Design review of the part built by this model. Coordinates are the model's own, in mm. A direction names the side the tool comes from. Coordinates: 2 decimals unless noted, no trailing zeros. Write item = value, one per line. Start each with the question number.
from build123d import *

# Parameters (mm, degrees)
F1_DEPTH     = 6
F3_DEPTH     = 5
F4_R         = 2.5
F5_DEPTH     = 28.0010001
F4_R_2       = 5
F6_DEPTH     = 6
F7_R         = 5
F8_DEPTH     = 7.7510001
F9_R         = 4.5
F10_DEPTH    = 1
F11_DEPTH    = 28.0010001
F12_T1_DEPTH = 5
F12_T3_DEPTH = 5.25
F13_R        = 0.5
F14_R        = 6
F14_R_2      = 4.5
F15_DEPTH    = 1.5


# Not quite as in the source:
# - a fillet or chamfer that OpenCascade refuses, or shapes differently, is made with other operations: its cross-section is extruded or revolved along the edge and cut away or added
# - a feature names something its author has since deleted; it is built from what else it names


with BuildPart() as f1:
    # F0 (on Top) → F1 (new body, symmetric)
    with BuildSketch(Plane.XY):
        with BuildLine():
            ThreePointArc((-3.75, -10.34105894), (1.2840732714, 10.9247954596), (1.25, -10.9287464972))
            Line((1.25, -10.9287464972), (1.25, -23.9287464972))
            Line((1.25, -23.9287464972), (6.25, -23.9287464972))
            Line((6.25, -23.9287464972), (6.25, -16.9424782941))
            add(Edge.make_bspline(
                [(13.9325423216, -1.3726851266), (12.6381972805, -10.4814385995), (6.7273111737, -10.6028057635), (6.25, -16.9424782941)],
                knots=[0, 0, 0, 0, 17.3620251065, 17.3620251065, 17.3620251065, 17.3620251065], degree=3))
            ThreePointArc((13.9325423216, -1.3726851266), (0.6871708294, 13.9831254107), (-14, 0))
            Line((-14, 0), (-14, -23.9287464972))
            Line((-14, -23.9287464972), (-3.75, -23.9287464972))
            Line((-3.75, -23.9287464972), (-3.75, -10.34105894))
        make_face()
    extrude(amount=F1_DEPTH, both=True)

    # F2 (on face) → F3 (join)
    with BuildSketch(Plane(origin=(-14, 0, 0), x_dir=(0, -1, 0), z_dir=(-1, 0, 0))):
        with BuildLine():
            ThreePointArc((35.9287464972, -6), (43.7069210902, -2.7781745931), (46.9287464972, 5))
            ThreePointArc((46.9287464972, 5), (38.4000033429, 15.7188100833), (26.0391302058, 9.8161695992))
            add(Edge.make_bspline(
                [(25.4869740085, 8.4596802299), (25.6594735822, 8.8218641875), (25.8423553432, 9.2659041852), (26.0391302058, 9.8161695992)],
                knots=[0.8880126886, 0.8880126886, 0.8880126886, 0.8880126886, 1, 1, 1, 1], degree=3))
            ThreePointArc((25.4869740085, 8.4596802299), (27.0108856963, -1.4398570431), (35.9287464972, -6))
        make_face()
        with BuildLine():
            add(Edge.make_bspline(
                [(25.4869740085, 8.4596802299), (25.6594735822, 8.8218641875), (25.8423553432, 9.2659041852), (26.0391302058, 9.8161695992)],
                knots=[0.8880126886, 0.8880126886, 0.8880126886, 0.8880126886, 1, 1, 1, 1], degree=3))
            ThreePointArc((26.0391302058, 9.8161695992), (25.7404513363, 9.1471245117), (25.4869740085, 8.4596802299))
        make_face()
        with BuildLine():
            Line((23.9287464972, 6), (23.9287464972, -6))
            Line((23.9287464972, -6), (35.9287464972, -6))
            ThreePointArc((35.9287464972, -6), (27.0108856963, -1.4398570431), (25.4869740085, 8.4596802299))
            add(Edge.make_bspline(
                [(19.1325701837, 6), (22.6899938416, 6), (23.8374523242, 6.4838968901), (24.9481407399, 7.3283338654), (25.4869740085, 8.4596802299)],
                knots=[0, 0, 0, 0, 0.5382002935, 0.8880126886, 0.8880126886, 0.8880126886, 0.8880126886], degree=3))
            Line((19.1325701837, 6), (23.9287464972, 6))
        make_face()
    extrude(amount=-F3_DEPTH)

    # F4 (on face) → F5 (cut, through all)
    with BuildSketch(Plane(origin=(-14, 0, 0), x_dir=(0, -1, 0), z_dir=(-1, 0, 0))):
        with Locations((17.34105894, 0)):
            Circle(F4_R)
    extrude(amount=-F5_DEPTH, mode=Mode.SUBTRACT)

    # F4 (on face) → F6 (cut)
    with BuildSketch(Plane(origin=(-14, 0, 0), x_dir=(0, -1, 0), z_dir=(-1, 0, 0))):
        with Locations((17.34105894, 0)):
            Circle(F4_R_2)
        with Locations((17.34105894, 0)):
            Circle(F4_R, mode=Mode.SUBTRACT)
    extrude(amount=-F6_DEPTH, mode=Mode.SUBTRACT)

    # F7 (on face) → F8 (cut, through all)
    with BuildSketch(Plane.YZ.offset(6.25)):
        with Locations((-17.34105894, 0)):
            Circle(F7_R)
    extrude(amount=F8_DEPTH, mode=Mode.SUBTRACT)

    # F9 (on face) → F10 (cut)
    with BuildSketch(Plane(origin=(-14, 0, 0), x_dir=(0, -1, 0), z_dir=(-1, 0, 0))):
        with BuildLine():
            ThreePointArc((34.4731002269, 12.6120689655), (28.5731123295, 2.5592734708), (39.3124481602, -1.9723068676))
            ThreePointArc((39.3124481602, -1.9723068676), (41.159616015, -2.0143070996), (41.6462424386, -0.231896421))
            ThreePointArc((41.6462424386, -0.231896421), (41.7469365287, -0.1196840486), (41.8454286992, -0.0055341094))
            ThreePointArc((41.8454286992, -0.0055341094), (43.5514595083, 0.7038684435), (43.2748339282, 2.5306884652))
            ThreePointArc((43.2748339282, 2.5306884652), (43.3214793257, 2.6740590451), (43.3653269111, 2.8183098875))
            ThreePointArc((43.3653269111, 2.8183098875), (44.6381060055, 4.1576479629), (43.6455935628, 5.7160805584))
            ThreePointArc((43.6455935628, 5.7160805584), (43.6302034221, 5.8660607565), (43.6118986313, 6.0157131902))
            ThreePointArc((43.6118986313, 6.0157131902), (44.2334947511, 7.7556589846), (42.6950381231, 8.7788619494))
            ThreePointArc((42.6950381231, 8.7788619494), (42.6202476169, 8.9097714466), (42.5429246828, 9.0392012737))
            ThreePointArc((42.5429246828, 9.0392012737), (42.4069051987, 10.8818330338), (40.58592621, 11.1946087142))
            ThreePointArc((40.58592621, 11.1946087142), (40.4645413227, 11.2840325668), (40.341439844, 11.3710781997))
            ThreePointArc((40.341439844, 11.3710781997), (39.4710946558, 13.0008917955), (37.6793899466, 12.5496852592))
            ThreePointArc((37.6793899466, 12.5496852592), (37.5321947731, 12.5823118919), (37.3843927675, 12.6120689655))
            ThreePointArc((37.3843927675, 12.6120689655), (35.9287464972, 13.75), (34.4731002269, 12.6120689655))
        make_face()
        with Locations((35.9287464972, 5)):
            Circle(F9_R, mode=Mode.SUBTRACT)
    extrude(amount=-F10_DEPTH, mode=Mode.SUBTRACT)

    # F11 (cut, through all): a face of the model
    f11_faces = [f1.faces().sort_by_distance(p)[0] for p in [
        (-14, -35.9287464972, 5),
    ]]
    extrude(f11_faces, amount=-F11_DEPTH, mode=Mode.SUBTRACT)

    # F12: fillet of radius 6 on 4 edges, made by hand

    # F12_s2 → F12_t1 (cut)
    with BuildSketch(Plane.YZ.offset(1.25)):
        with BuildLine():
            ThreePointArc((-17.9287464972, -6), (-22.1713871843, -4.2426406871), (-23.9287464972, 0))
            Line((-23.9287464972, 0), (-24.0487464972, 0))
            Line((-24.0487464972, 0), (-24.0487464972, -6.12))
            Line((-24.0487464972, -6.12), (-17.9287464972, -6.12))
            Line((-17.9287464972, -6.12), (-17.9287464972, -6))
        make_face()
        with BuildLine():
            ThreePointArc((-17.9287464972, 6), (-22.1713871843, 4.2426406871), (-23.9287464972, 0))
            Line((-23.9287464972, 0), (-24.0487464972, 0))
            Line((-24.0487464972, 0), (-24.0487464972, 6.12))
            Line((-24.0487464972, 6.12), (-17.9287464972, 6.12))
            Line((-17.9287464972, 6.12), (-17.9287464972, 6))
        make_face()
    extrude(amount=F12_T1_DEPTH, mode=Mode.SUBTRACT)

    # F12_s4 → F12_t3 (cut)
    with BuildSketch(Plane.YZ.offset(-9)):
        with BuildLine():
            ThreePointArc((-17.9287464972, -6), (-22.1713871843, -4.2426406871), (-23.9287464972, 0))
            Line((-23.9287464972, 0), (-24.0487464972, 0))
            Line((-24.0487464972, 0), (-24.0487464972, -6.12))
            Line((-24.0487464972, -6.12), (-17.9287464972, -6.12))
            Line((-17.9287464972, -6.12), (-17.9287464972, -6))
        make_face()
        with BuildLine():
            ThreePointArc((-17.9287464972, 6), (-22.1713871843, 4.2426406871), (-23.9287464972, 0))
            Line((-23.9287464972, 0), (-24.0487464972, 0))
            Line((-24.0487464972, 0), (-24.0487464972, 6.12))
            Line((-24.0487464972, 6.12), (-17.9287464972, 6.12))
            Line((-17.9287464972, 6.12), (-17.9287464972, 6))
        make_face()
    extrude(amount=F12_T3_DEPTH, mode=Mode.SUBTRACT)

    # F13
    f13_edges = [f1.edges().sort_by_distance(p)[0] for p in [
        (6.25, -22.171387, 4.242641),
        (6.25, -17.435612, -6),
        (10.470288, -9.384464, -6),
        (6.25, -17.435612, 6),
        (10.470288, -9.384464, 6),
        (0.687171, 13.983125, -6),
        (0.687171, 13.983125, 6),
        (-14, -17.964373, -6),
        (-14, -44.846607, 11.439857),
        (-14, -22.786929, 6.220362),
        (-14, -9.566285, 6),
    ]]
    fillet(f13_edges, radius=F13_R)

    # F14 (on face) → F15 (cut)
    with BuildSketch(Plane.YZ.offset(-9)):
        with Locations((-35.9287464972, 5)):
            Circle(F14_R)
        with Locations((-35.9287464972, 5)):
            Circle(F14_R_2, mode=Mode.SUBTRACT)
    extrude(amount=-F15_DEPTH, mode=Mode.SUBTRACT)


solid = f1.part
Q1. To check wall thickness, follow line 1 (X direction, y = -37, z = 15.25); line 2 (X direction, y = -35.5, z = -0.75); line 3 (X direction, y = 6.5, z = 2.75). State the ranges of each line that lie inside material, in increasing order. Write a range as from..to.
Q2. For faces 1 (the face through (-3.75, -14, 0)), 2 (the face through (-13.51, -35.96, 13.75)), 3 (the face through (-6, -10, 6)), list the 3-axis set-ups (+Z, -Z, +X, -X, +Y, -Y) from which the entire face can be reached by the end or side of a thin tool; tool diameter is ignored.
Q3. Mouldability with a two-part tool opening along X and no side actions: class faces 4 (the face through (-8, -19.5, -2.2)), 5 (the face through (0.838, 10.968, 0.084)), 6 (the face through (-13.507, -28.517, 2.735)) as released by +X, released by -X, zero draft, split by the parting line, or undercut.
Q4. Clearance check with flat-ended pins moving along their axes: P1, Ø5.5, axis at y = -35.93, z = 5, coming from the +X side; P2, Ø9.5, axis at y = -33, z = 3.5, coming from the +X side; P3, Ø8, axis at y = -17.34, z = 0, coming from the +X side; P4, Ø6, axis at y = -14, z = -2, coming from the +X side. State where each tip first meets the part, or that it passes through.
Values follow:
q1.line_1 = -14..-9
q1.line_2 = -13..-10.5
q1.line_3 = -12.4..-8.87, 8.87..12.4
q2.face_1 = +Z, -Z, -Y
q2.face_2 = -X
q2.face_3 = +Z, +X, -X, +Y
q3.face_4 = released by -X
q3.face_5 = undercut
q3.face_6 = zero draft
q4.P1 = through
q4.P2 = -9
q4.P3 = 6.25
q4.P4 = 9.08
